The listing builds one solid part. Answer for the finished solid, in the listing's coordinates (mm). A direction names the side the tool comes from. Give positions to 0.01 mm unless a question says otherwise; leave off trailing zeros. One line per item, written item: value. Start each with the question number.
Q1. A cutting plane is placed at A-A, the plane z = 10. State how many separate pieces and enclosed holes the cut face has, and give its area (3 significant figures).
Q2. For faces 1 (the cylindrical face through (8.301, 7.715, 9.673)), 2 (the flat face through (-11.268, 1.851, 6.854)), 3 (the cylindrical face through (11.27, 0.12, 13.75)), 4 (the flat face through (-2, 2, 25.5)), 5 (the cylindrical face through (-8.301, -7.715, 9.673)), determine the directions among +Z, -Z, +X, -X, +Y, -Y from which every point of the face is accessible in a straight line to the end or side of a thin tool.
Q3. Consider L1, parallel to X at y = 3.5, z = 5; L2, parallel to Y at x = 0, z = 27.3; L3, parallel to X at y = 0, z = 23.25. Determine where each line is inside the solid, lowest interval first.
Q4. The mould has two halves that part along Z. Classify faces 6 (the cylindrical face through (-10.23, 4.06, 0.86)), 7 (the flat face through (11.27, 1.95, 6.49)), 8 (the cylindrical face through (12.199, 7.715, 14.712)), 9 (the cylindrical face through (-11.07, 0.1, 28.5)): +Z half, -Z half, draft (parallel to the pull), parting line (faces both ways), or undercut.
Q5. Flat-ended cylindrical pins translate along their axes: pin 1 (6 mm diameter, centred on y = 0, z = 10, fed in from +X); pin 2 (4.5 mm diameter, centred on x = 0, y = 0, fed in from +Z); pin 3 (8 mm diameter, centred on x = 1, y = -1, fed in from -Z) (3 decimals); pin 4 (0.9 mm diameter, centred on x = -9, y = 0, fed in from +Z). Find the tip coordinate at first contact, or state that the pin passes through.
from build123d import *

# Parameters (mm, degrees)
CROQUIS1_W                   = 25
CROQUIS1_H                   = 20
SALIENTE_EXTRUIR1_DEPTH      = 30
CORTAR_EXTRUIR1_REACH        = 40.161
CROQUIS2_W                   = 16
CROQUIS2_H                   = 45
TALADRO_DE_MARGEN_PARA_M51_D = 4.6
CROQUIS8_R                   = 3.75
CORTAR_EXTRUIR4_DEPTH        = 2.5
CORTAR_EXTRUIR5_DEPTH        = 2.5
TALADRO_DE_MARGEN_PARA_M52_D = 4.8
CORTAR_EXTRUIR6_DEPTH        = 3
REDONDEO1_R                  = 10
REDONDEO2_R                  = 5
REDONDEO3_R                  = 8
CORTAR_EXTRUIR7_DEPTH        = 39.810436741
CORTAR_EXTRUIR8_DEPTH        = 2.5
CORTAR_EXTRUIR9_START        = -10
CORTAR_EXTRUIR9_DEPTH        = 2
CORTAR_EXTRUIR9_START_2      = 8
CORTAR_EXTRUIR9_2_DEPTH      = 2
REDONDEO4_R                  = 2
REDONDEO5_R                  = 1


# Read off the part's stored shape, not the designer's step: Cortar-Extruir9
# Some blends are built 0.0001 mm under size
with BuildPart() as part:
    # Croquis1 → Saliente-Extruir1 (new body)
    with BuildSketch(Plane.XY):
        Rectangle(CROQUIS1_W, CROQUIS1_H)
    extrude(amount=SALIENTE_EXTRUIR1_DEPTH)

    # Croquis2 → Cortar-Extruir1 (cut, up to next)
    with BuildSketch(Plane(origin=(0, 10, 0), x_dir=(1, 0, 0), z_dir=(0, 1, 0)), mode=Mode.PRIVATE) as cortar_extruir1_sk1:
        Rectangle(CROQUIS2_W, CROQUIS2_H)
    cortar_extruir1_tool1 = extrude(cortar_extruir1_sk1.sketch, amount=-CORTAR_EXTRUIR1_REACH, mode=Mode.PRIVATE) & part.part
    add(cortar_extruir1_tool1.solids().sort_by_distance((0, 10, 0))[0], mode=Mode.SUBTRACT)

    # Taladro de margen para M51 (through all)
    with Locations(Plane(origin=(12.5, 0, 0), x_dir=(0, 0, -1), z_dir=(1, 0, 0))):
        with Locations((-10, 0)):
            Hole(TALADRO_DE_MARGEN_PARA_M51_D / 2)

    # Croquis8 → Cortar-Extruir4 (cut)
    with BuildSketch(Plane(origin=(12.5, 0, 0), x_dir=(0, 0, -1), z_dir=(1, 0, 0))):
        with Locations((-10, 0)):
            Circle(CROQUIS8_R)
    extrude(amount=-CORTAR_EXTRUIR4_DEPTH, mode=Mode.SUBTRACT)

    # Croquis9 → Cortar-Extruir5 (cut)
    with BuildSketch(Plane.ZY.offset(12.5)):
        Polygon((5.785343035, 0), (7.892671517, -3.65), (12.107328483, -3.65), (14.214656965, 0), (12.107328483, 3.65), (7.892671517, 3.65), align=None)
    extrude(amount=-CORTAR_EXTRUIR5_DEPTH, mode=Mode.SUBTRACT)

    # Taladro de margen para M52 (through all)
    with Locations(Plane.XY.offset(30)):
        with Locations((0, 0)):
            Hole(TALADRO_DE_MARGEN_PARA_M52_D / 2)

    # Croquis13 → Cortar-Extruir6 (cut)
    with BuildSketch(Plane(origin=(0, 0, 22.5), x_dir=(-1, 0, 0), z_dir=(0, 0, -1))):
        Polygon((2.109650745, 3.648658256), (-2.105005367, 3.651340266), (-4.214656112, 0.00268201), (-2.109650745, -3.648658256), (2.105005367, -3.651340266), (4.214656112, -0.00268201), align=None)
    extrude(amount=-CORTAR_EXTRUIR6_DEPTH, mode=Mode.SUBTRACT)

    # Redondeo1
    redondeo1_edges = [part.edges().sort_by_distance(p)[0] for p in [
        (-10.25, -10, 0),
        (-10.25, 10, 0),
        (10.25, -10, 0),
        (10.25, 10, 0),
    ]]
    fillet(redondeo1_edges, radius=REDONDEO1_R - 0.0001)  # a hair under: the kernel refuses the full size

    # Redondeo2
    redondeo2_edges = [part.edges().sort_by_distance(p)[0] for p in [
        (-12.5, 0, 30),
        (12.5, 0, 30),
    ]]
    fillet(redondeo2_edges, radius=REDONDEO2_R)

    # Redondeo3
    # the kernel refuses this fillet: 8 mm, written as the material it adds along each edge
    with BuildSketch(Plane(origin=(-8, 10, 22.5), x_dir=(0, 0, -1), z_dir=(0, -1, 0))) as redondeo3_piece_1_section:
        with BuildLine():
            CenterArc((REDONDEO3_R, REDONDEO3_R), REDONDEO3_R, 180, 90)
            Line((0, REDONDEO3_R), (0, 0))
            Line((0, 0), (REDONDEO3_R, 0))
        make_face()
    redondeo3_piece_1 = extrude(amount=40, mode=Mode.PRIVATE)
    redondeo3_piece_1 = split(redondeo3_piece_1, bisect_by=Plane(origin=(-1.542701741, 4.632087449, 20.877990823), z_dir=(-0.8663434050364778, 0.49944880072916537, 0)), keep=Keep.TOP, mode=Mode.PRIVATE)
    add(redondeo3_piece_1)
    with BuildSketch(Plane(origin=(-8, 30, 22.5), x_dir=(0, 0, -1), z_dir=(0, -1, 0))) as redondeo3_piece_2_section:
        with BuildLine():
            CenterArc((REDONDEO3_R, REDONDEO3_R), REDONDEO3_R, 180, 90)
            Line((0, REDONDEO3_R), (0, 0))
            Line((0, 0), (REDONDEO3_R, 0))
        make_face()
    redondeo3_piece_2 = extrude(amount=60, mode=Mode.PRIVATE)
    redondeo3_piece_2 = split(redondeo3_piece_2, bisect_by=Plane(origin=(-1.583425809, 4.561447519, 22.44370091), z_dir=(0.8663434050364778, -0.49944880072916537, 0)), keep=Keep.TOP, mode=Mode.PRIVATE)
    redondeo3_piece_2 = split(redondeo3_piece_2, bisect_by=Plane(origin=(-1.267040589, 3.649194454, 22.44370091), z_dir=(-0.0006363531971100188, 0.9999997975272839, 0)), keep=Keep.TOP, mode=Mode.PRIVATE)
    add(redondeo3_piece_2)
    with BuildSketch(Plane(origin=(-8, 30, 22.5), x_dir=(0, 0, -1), z_dir=(0, -1, 0))) as redondeo3_piece_3_section:
        with BuildLine():
            CenterArc((REDONDEO3_R, REDONDEO3_R), REDONDEO3_R, 180, 90)
            Line((0, REDONDEO3_R), (0, 0))
            Line((0, 0), (REDONDEO3_R, 0))
        make_face()
    redondeo3_piece_3 = extrude(amount=40, mode=Mode.PRIVATE)
    redondeo3_piece_3 = split(redondeo3_piece_3, bisect_by=Plane(origin=(-1.265169081, -3.650805834, 22.443951569), z_dir=(0.0006363531971099136, -0.9999997975272839, 0)), keep=Keep.TOP, mode=Mode.PRIVATE)
    add(redondeo3_piece_3)
    with BuildSketch(Plane(origin=(-8, 30, 22.5), x_dir=(0, 0, -1), z_dir=(0, -1, 0))) as redondeo3_piece_4_section:
        with BuildLine():
            CenterArc((REDONDEO3_R, REDONDEO3_R), REDONDEO3_R, 180, 90)
            Line((0, REDONDEO3_R), (0, 0))
            Line((0, 0), (REDONDEO3_R, 0))
        make_face()
    redondeo3_piece_4 = extrude(amount=60, mode=Mode.PRIVATE)
    redondeo3_piece_4 = split(redondeo3_piece_4, bisect_by=Plane(origin=(-3.239385645, -1.689420276, 21.740409099), z_dir=(-0.865707051839368, -0.5005509967981187, 0)), keep=Keep.TOP, mode=Mode.PRIVATE)
    redondeo3_piece_4 = split(redondeo3_piece_4, bisect_by=Plane(origin=(-4.581718949, -3.652916331, 21.740409099), z_dir=(-0.0006363531971099136, 0.9999997975272839, 0)), keep=Keep.TOP, mode=Mode.PRIVATE)
    add(redondeo3_piece_4)
    with BuildSketch(Plane(origin=(8, 10, 22.5), x_dir=(-1, 0, 0), z_dir=(0, -1, 0))) as redondeo3_piece_5_section:
        with BuildLine():
            CenterArc((REDONDEO3_R, REDONDEO3_R), REDONDEO3_R, 180, 90)
            Line((0, REDONDEO3_R), (0, 0))
            Line((0, 0), (REDONDEO3_R, 0))
        make_face()
    redondeo3_piece_5 = extrude(amount=40, mode=Mode.PRIVATE)
    redondeo3_piece_5 = split(redondeo3_piece_5, bisect_by=Plane(origin=(1.539300271, 4.629731866, 20.879744511), z_dir=(0.8657070518393678, 0.5005509967981188, 0)), keep=Keep.TOP, mode=Mode.PRIVATE)
    add(redondeo3_piece_5)
    with BuildSketch(Plane(origin=(8, 30, 22.5), x_dir=(-1, 0, 0), z_dir=(0, -1, 0))) as redondeo3_piece_6_section:
        with BuildLine():
            CenterArc((REDONDEO3_R, REDONDEO3_R), REDONDEO3_R, 180, 90)
            Line((0, REDONDEO3_R), (0, 0))
            Line((0, 0), (REDONDEO3_R, 0))
        make_face()
    redondeo3_piece_6 = extrude(amount=60, mode=Mode.PRIVATE)
    redondeo3_piece_6 = split(redondeo3_piece_6, bisect_by=Plane(origin=(1.579702806, 4.559855351, 22.443951569), z_dir=(-0.8657070518393678, -0.5005509967981188, 0)), keep=Keep.TOP, mode=Mode.PRIVATE)
    redondeo3_piece_6 = split(redondeo3_piece_6, bisect_by=Plane(origin=(1.265169081, 3.650805834, 22.443951569), z_dir=(-0.0006363531971100188, 0.9999997975272839, 0)), keep=Keep.TOP, mode=Mode.PRIVATE)
    add(redondeo3_piece_6)
    with BuildSketch(Plane(origin=(8, 30, 22.5), x_dir=(-1, 0, 0), z_dir=(0, -1, 0))) as redondeo3_piece_7_section:
        with BuildLine():
            CenterArc((REDONDEO3_R, REDONDEO3_R), REDONDEO3_R, 180, 90)
            Line((0, REDONDEO3_R), (0, 0))
            Line((0, 0), (REDONDEO3_R, 0))
        make_face()
    redondeo3_piece_7 = extrude(amount=40, mode=Mode.PRIVATE)
    redondeo3_piece_7 = split(redondeo3_piece_7, bisect_by=Plane(origin=(3.24131014, -1.685682967, 21.739264783), z_dir=(0.8663434050364778, -0.49944880072916537, 0)), keep=Keep.TOP, mode=Mode.PRIVATE)
    add(redondeo3_piece_7)
    with BuildSketch(Plane(origin=(8, 30, 22.5), x_dir=(-1, 0, 0), z_dir=(0, -1, 0))) as redondeo3_piece_8_section:
        with BuildLine():
            CenterArc((REDONDEO3_R, REDONDEO3_R), REDONDEO3_R, 180, 90)
            Line((0, REDONDEO3_R), (0, 0))
            Line((0, 0), (REDONDEO3_R, 0))
        make_face()
    redondeo3_piece_8 = extrude(amount=60, mode=Mode.PRIVATE)
    redondeo3_piece_8 = split(redondeo3_piece_8, bisect_by=Plane(origin=(1.267040588, -3.649194454, 22.44370091), z_dir=(0.0006363531971099136, -0.9999997975272839, 0)), keep=Keep.TOP, mode=Mode.PRIVATE)
    redondeo3_piece_8 = split(redondeo3_piece_8, bisect_by=Plane(origin=(1.583425809, -4.561447518, 22.44370091), z_dir=(-0.8663434050364778, 0.49944880072916537, 0)), keep=Keep.TOP, mode=Mode.PRIVATE)
    add(redondeo3_piece_8)

    # Croquis14 → Cortar-Extruir7 (cut, through all)
    with BuildSketch(Plane.ZY.offset(10)):
        Polygon((8.558178994, 1.791968801), (7.1476261, 0.592860429), (7.1476261, -0.592860429), (8.558178994, -1.791968801), align=None)
    extrude(amount=-CORTAR_EXTRUIR7_DEPTH, mode=Mode.SUBTRACT)

    # Croquis15 → Cortar-Extruir8 (cut)
    with BuildSketch(Plane(origin=(12.5, 0, 0), x_dir=(0, 0, -1), z_dir=(1, 0, 0))):
        with BuildLine():
            Line((-7.589546464, 2.872666662), (-5.357789242, 1))
            Line((-5.357789242, 1), (-5.357789242, -1))
            Line((-5.357789242, -1), (-7.589546464, -2.872666662))
            ThreePointArc((-7.589546464, -2.872666662), (-6.25, 0), (-7.589546464, 2.872666662))
        make_face()
    extrude(amount=-CORTAR_EXTRUIR8_DEPTH, mode=Mode.SUBTRACT)

    # Cortar-Extruir9 outline → Cortar-Extruir9 (cut)
    with BuildSketch(Plane(origin=(0, 0, 0), x_dir=(1, 0, 0), z_dir=(0, 1, 0)).offset(CORTAR_EXTRUIR9_START)):
        with BuildLine():
            Line((12.5, -25), (12.5, -3))
            Line((12.5, -3), (8, -3))
            Line((8, -3), (8, -14.5))
            ThreePointArc((8, -14.5), (5.656854249, -20.156854249), (0, -22.5))
            ThreePointArc((0, -22.5), (-5.656854249, -20.156854249), (-8, -14.5))
            Line((-8, -14.5), (-8, -3))
            Line((-8, -3), (-12.5, -3))
            Line((-12.5, -3), (-12.5, -25))
            ThreePointArc((-12.5, -25), (-11.035533906, -28.535533906), (-7.5, -30))
            Line((-7.5, -30), (7.5, -30))
            ThreePointArc((7.5, -30), (11.035533906, -28.535533906), (12.5, -25))
        make_face()
    extrude(amount=CORTAR_EXTRUIR9_DEPTH, mode=Mode.SUBTRACT)

    # Cortar-Extruir9 2 outline → Cortar-Extruir9 2 (cut)
    with BuildSketch(Plane(origin=(0, 0, 0), x_dir=(1, 0, 0), z_dir=(0, 1, 0)).offset(CORTAR_EXTRUIR9_START_2)):
        with BuildLine():
            Line((12.5, -25), (12.5, -3))
            Line((12.5, -3), (8, -3))
            Line((8, -3), (8, -14.5))
            ThreePointArc((8, -14.5), (5.656854249, -20.156854249), (0, -22.5))
            ThreePointArc((0, -22.5), (-5.656854249, -20.156854249), (-8, -14.5))
            Line((-8, -14.5), (-8, -3))
            Line((-8, -3), (-12.5, -3))
            Line((-12.5, -3), (-12.5, -25))
            ThreePointArc((-12.5, -25), (-11.035533906, -28.535533906), (-7.5, -30))
            Line((-7.5, -30), (7.5, -30))
            ThreePointArc((7.5, -30), (11.035533906, -28.535533906), (12.5, -25))
        make_face()
    extrude(amount=CORTAR_EXTRUIR9_2_DEPTH, mode=Mode.SUBTRACT)

    # Redondeo4
    redondeo4_edges = [part.edges().sort_by_distance(p)[0] for p in [
        (-10.25, 8, 3.999933333),
        (10.25, 8, 3.999933333),
        (10.25, -8, 3.999933333),
        (-10.25, -8, 3.999933333),
    ]]
    fillet(redondeo4_edges, radius=REDONDEO4_R)

    # Redondeo5
    redondeo5_edges = [part.edges().sort_by_distance(p)[0] for p in [
        (-5.656854249, 8, 20.156854249),
        (12.5, 8, 14.854217587),
        (11.035533906, 8, 28.535533906),
        (-11.035533906, 8, 28.535533906),
        (-12.5, 8, 14.854217587),
        (5.656854249, 8, 20.156854249),
        (8, 8, 9.604217587),
        (0, 8, 30),
        (-5.656854249, -8, 20.156854249),
        (11.035533906, -8, 28.535533906),
        (-11.035533906, -8, 28.535533906),
        (5.656854249, -8, 20.156854249),
        (-8, -8, 9.604217587),
        (0, -8, 30),
        (-12.5, -8, 14.854217587),
        (8, -8, 9.604217587),
        (12.5, -8, 14.854217587),
        (12.5, -4.114415603, 0.885603147),
        (12.5, 7.870827023, 4.001323974),
        (12.5, -7.870827023, 4.001323974),
        (8, 4.114415603, 0.885603147),
        (8, 7.870827023, 4.001323974),
        (8, -7.870827023, 4.001323974),
        (-8, -4.114415603, 0.885603147),
        (-8, 8, 9.604217587),
        (-8, 7.870827023, 4.001323974),
        (-8, -7.870827023, 4.001323974),
        (-12.5, 4.114415603, 0.885603147),
        (-12.5, 7.870827023, 4.001323974),
        (-12.5, -7.870827023, 4.001323974),
        (-8, 4.114415603, 0.885603147),
        (-12.5, -4.114415603, 0.885603147),
        (12.5, 4.114415603, 0.885603147),
        (8, -4.114415603, 0.885603147),
    ]]
    fillet(redondeo5_edges, radius=REDONDEO5_R)


solid = part.part
Answer block:
1. separate pieces: 4
1. enclosed holes: 0
1. area: 86.9 mm^2
2. face 1: -Z, +Y
2. face 2: -X
2. face 3: +X
2. face 4: -Z
2. face 5: -Z, -Y
3. L1: -12.5 to -8, 8 to 12.5
3. L2: -8 to -2.4, 2.4 to 8
3. L3: -12.5 to -4.21, 4.21 to 12.5
4. face 6: -Z half
4. face 7: undercut
4. face 8: draft
4. face 9: +Z half
5. pin 1: x = 10
5. pin 2: through
5. pin 3: z = 20.745
5. pin 4: z = 29.89
